The listing builds one solid part. Answer for the finished solid, in the listing's coordinates (mm). Face numbers are marked on the shaded views. A direction names the side the tool comes from. Coordinates: 2 decimals unless noted, no trailing zeros. Loops run counter-clockwise (first coordinate to the right, second up) from the corner with the lowest first, then second, coordinate; pieces in that order, holes last. Notation, with made-up numbers: (30.25, 26.5) - (76.25, 26.5) arc R15 ccw to (76.25, 34.5) - close; hole circle Ø5 at (56.5, 89.5). An arc over 180 degrees is marked (long way). Return JSON: item names as keys, results as strings. Group by question number.
1. The mould has two halves that part along X. Classify the marked faces 3, 4, 5 and 6: pulls with the +X half, pulls with the -X half, needs draft (parallel to the pull), parting line crosses it, or undercut.
2. Each of these flat-tipped pins is pushed along its axis until it touches: P1, Ø7.5, axis at x = -8, z = 12, coming from the -Y side; P2, Ø1.5, axis at x = 9, y = 2.5, coming from the -Z side; P3, Ø7, axis at x = 0, z = 0, coming from the -Y side; P4, Ø4, axis at y = 1.5, z = 8.5, coming from the +X side. Where does it stop, or does it pass through?
3. Section D-D (z = -10.16) is taken. Write down the section's boundary in (x, y) (3 decimals), and give its area (3 significant figures).
4. Find the intervals of material crossed by line 1 along X through (y, z) = (4, 0) (3 decimals); line 2 along X through (y, z) = (4.5, 7); line 3 along Z through (x, y) = (1, 7.25), in increasing order.
5. Section B-B (y = 2.5) is taken. Write down the section's boundary in (x, z) (3 decimals), and give its area (3 significant figures).
6. Which of the six approach directions +Z, -Z, +X, -X, +Y, -Y give full straight-line access (tool end or side, diameter ignored) to the marked faces 1 and 2?
7. Section C-C (x = 0) is taken. Write down the section's boundary in (y, z) (3 decimals), and give its area (3 significant figures).
8. Section A-A (z = 0) is taken. Write down the section's boundary in (x, y) (3 decimals).
Autodesk Inventor part; units mm, degrees
ref_plane "YZ Plane" through (0, 0, 0) normal (1, 0, 0) x (0, 1, 0)
ref_plane "XZ Plane" through (0, 0, 0) normal (0, 1, 0) x (-1, 0, 0)
ref_plane "XY Plane" through (0, 0, 0) normal (0, 0, 1) x (1, 0, 0)
sketch "Sketch1" plane through (0, 0, 0) normal (0, 1, 0) x (-1, 0, 0)
  circle A0 centre (0, 0) radius 3.81
  circle A1 centre (0, 0) radius 16.51
  line L0 (0, 0) -> (10.16, 0)
  line L1 (0, 0) -> (-10.16, 0)
  circle A2 centre (10.16, 0) radius 1.524
  circle A3 centre (-10.16, 0) radius 1.524
  circle A4 centre (0, 0) radius 5.0292
  circle A5 centre (0, 0) radius 15.2908
  line L2 (0, 0) -> (0, 10.16)
  circle A6 centre (0, 10.16) radius 2.3812
  line L3 (0, 0) -> (2.5146, 4.3554)
  line L4 (0, 0) -> (5.0292, 0) construction
  line L5 (2.5146, 4.3554) -> (7.6454, 13.2422)
  line L6 (0, 0) -> (-2.5146, 4.3554)
  line L7 (-2.5146, 4.3554) -> (-7.6454, 13.2422)
  line L8 (0, 0) -> (2.5146, -4.3554)
  line L9 (2.5146, -4.3554) -> (7.6454, -13.2422)
  line L10 (0, 0) -> (-2.5146, -4.3554)
  line L11 (-2.5146, -4.3554) -> (-7.6454, -13.2422)
  line L12 (0.4064, 16.8443) -> (-0.4064, 16.8443)
  line L13 (-0.4064, 16.8443) -> (-0.4064, 15.0672)
  line L14 (-0.4064, 15.0672) -> (0.4064, 15.0672)
  line L15 (0.4064, 15.0672) -> (0.4064, 16.8443)
  line L16 (0.4064, 16.8443) -> (-0.4064, 15.0672) construction
  line L17 (-0.4064, 16.8443) -> (0.4064, 15.0672) construction
  line L18 (0.4064, -15.0362) -> (-0.4064, -15.0362)
  line L19 (-0.4064, -15.0362) -> (-0.4064, -16.8142)
  line L20 (-0.4064, -16.8142) -> (0.4064, -16.8142)
  line L21 (0.4064, -16.8142) -> (0.4064, -15.0362)
  line L22 (0.4064, -15.0362) -> (-0.4064, -16.8142) construction
  line L23 (-0.4064, -15.0362) -> (0.4064, -16.8142) construction
  circle A7 centre (0, 10.16) radius 1.524
  line L24 (0, 0) -> (0, -10.16)
  circle A8 centre (0, -10.16) radius 1.524
  circle A9 centre (0, 0) radius 0.7937
  line L25 (0, 0) -> (-13.5242, 9.4697)
  line L26 (0, 0) -> (16.51, 0) construction
  line L27 (-13.9904, 8.8039) -> (-0.408, -0.7066)
  line L28 (-13.058, 10.1356) -> (0.2563, 0.8128)
  line L29 (16.49, 0.8128) -> (16.51, 0.8128)
  line L30 (16.49, -0.8128) -> (16.51, -0.8128)
  line L31 (0, 0) -> (-0.408, -0.7066)
  line L32 (0.2563, 0.8128) -> (0.408, 0.7066)
  line L33 (0, 0) -> (0.408, 0.7066)
  line L34 (-13.058, 10.1356) -> (-13.9904, 8.8039)
  line L35 (0.408, 0.7066) -> (-0.408, -0.7066)
  line L36 (-7.6454, 13.2422) -> (-8.255, 14.2981)
  line L37 (7.6454, 13.2422) -> (8.255, 14.2981)
  line L38 (-7.6454, -13.2422) -> (-8.255, -14.2981)
  line L39 (7.6454, -13.2422) -> (8.255, -14.2981)
  line L40 (0, 0) -> (13.2422, 7.6454)
  line L41 (13.2422, 7.6454) -> (14.2981, 8.255)
  line L42 (0, 0) -> (-13.2422, -7.6454)
  line L43 (-13.2422, -7.6454) -> (-14.2981, -8.255)
  point P0 (0, 15.9557)
  point P1 (0, -15.9252)
  point P2 (-13.974, 8.7925)
  point P3 (-1.4171, 0)
  point P4 (-0.7937, 0)
  point P5 (-0.3969, 0.6874)
  point P6 (-0.9616, 1.6656)
  point P7 (-13.0416, 10.1241)
  point P8 (1.905, 3.2996)
  point P9 (-1.905, 3.2996)
  point P10 (1.905, -3.2996)
  point P11 (-1.905, -3.2996)
  point P12 (4.3554, 2.5146)
  point P13 (-4.3554, -2.5146)
  point P14 (3.2996, 1.905)
  point P15 (-3.2996, -1.905)
  dimension "d1" = 33.02
  dimension "d0" = 7.62
  dimension "d2" = 10.16
  dimension "d3" = 10.16
  dimension "d4" = 3.048
  dimension "d5" = 3.048
  dimension "d8" = 10.0584
  dimension "d9" = 30.5816
  dimension "d10" = 10.16
  dimension "d11" = 4.7625
  dimension "d12" = 60
  dimension "d17" = 0.8128
  dimension "d18" = 0.8128
  dimension "d19" = 1.778
  dimension "d24" = 3.048
  dimension "d25" = 10.16
  dimension "d26" = 3.048
  dimension "d41" = 1.5875
  dimension "d42" = 145
  dimension "d43" = 0.8128
  dimension "d44" = 0.8128
extrude "Extrusion1" add sketch "Sketch1" along normal blind 7.5184 contours L0 A4 L8 A0 | A0 L40 A4 L0 | A0 L3 A4 L40 | L8 A4 L24 A0 | A2 | A4 L40 A5 L9 | A0 L2 A4 L3 | A4 L5 A5 L40 | L24 A4 L10 A0 | A8 | L9 A5 L21 L18 L19 L11 A4 | A0 L6 A4 L2 | A7 | A6 | A4 L7 A5 L13 L14 L15 L5 | L41 A1 L39 A5 | A5 L37 A1 L41 | L10 A4 L42 A0 | L39 A1 L21 A5 | A0 L28 A4 L6 | A5 L15 A1 L37 | L42 A4 L1 A0 | L11 A5 L42 A4 | L21 A1 L19 A5 | A5 L19 L18 L21 | L25 A4 L28 A0 | A0 L27 A4 L25 | A4 L28 A5 L7 | L15 L14 L13 A5 | A5 L13 A1 L15 | L1 A4 L27 A0 | A3 | L42 A5 L27 A4 | L38 A1 L43 A5 | A5 L19 A1 L38 | L25 A5 L28 A4 | A4 L27 A5 L25 | L36 A1 L13 A5 | A5 L28 A1 L36 | L43 A1 L27 A5 | L25 A1 L28 A5 | A5 L27 A1 L25
extrude "Extrusion2" cut sketch "Sketch1" along normal blind 6.35 contours A0 L3 A4 L40 | A0 L2 A4 L3 | A4 L5 A5 L40 | A0 L6 A4 L2 | A7 | A6 | A4 L7 A5 L13 L14 L15 L5 | A5 L37 A1 L41 | A5 L15 A1 L37 | L15 L14 L13 A5 | A5 L13 A1 L15 | L36 A1 L13 A5
extrude "Extrusion3" cut sketch "Sketch1" along normal blind 6.35 contours L8 A4 L24 A0 | L24 A4 L10 A0 | A8 | L9 A5 L21 L18 L19 L11 A4 | L10 A4 L42 A0 | L39 A1 L21 A5 | L11 A5 L42 A4 | L21 A1 L19 A5 | A5 L19 L18 L21 | L38 A1 L43 A5 | A5 L19 A1 L38
extrude "Extrusion6" cut sketch "Sketch1" along normal blind 7.5184 contours L1 L27 A0 L25 A9 | A9 L25 A0 L28 L6 | L25 A4 L28 A0 | A0 L27 A4 L25 | L25 A5 L28 A4 | A4 L27 A5 L25 | L25 A1 L28 A5 | A5 L27 A1 L25
hole "Hole3" at (10.16, 0, 0) direction (0, 1, 0) diameter 3.81 end through all
hole "Hole4" at (-10.16, 0, 0) direction (0, 1, 0) diameter 3.81 end through all
hole "Hole5" at (0, 0, -10.16) direction (0, 1, 0) diameter 3.81 end through all
hole "Hole6" at (0, 0, 10.16) direction (0, 1, 0) diameter 3.81 end through all
properties part number "tab3"
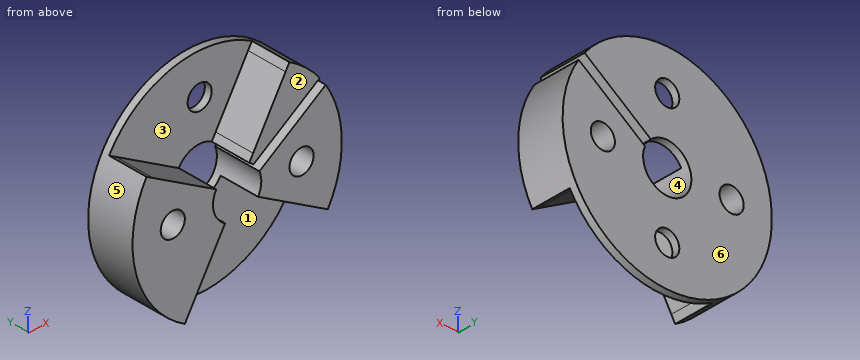
The answers:
{
 "1": {"face 3": "undercut", "face 4": "undercut", "face 5": "parting line crosses it", "face 6": "needs draft"},
 "2": {"P1": "stops at y = 6.35", "P2": "stops at z = -5.63", "P3": "passes through", "P4": "stops at x = 15.18"},
 "3": {"outline": "(-13.014, 0) - (-5.866, 0) - (-5.866, 6.35) - (-1.905, 6.35) - (-1.905, 7.518) - (-13.014, 7.518) - close; (1.905, 6.35) - (13.014, 6.35) - (13.014, 7.518) - (1.905, 7.518) - close", "area": "71.3 mm2"},
 "4": {"line 1": "x = -16.51 to -12.065, -8.255 to -3.81, 3.81 to 8.255, 12.065 to 16.51", "line 2": "x = -14.95 to -12.12, 4.04 to 8.58, 11.41 to 14.95", "line 3": "z = -16.48 to -11.78, -8.54 to -3.68, 3.68 to 8.54, 11.78 to 16.48"},
 "5": {"outline": "(-14.298, 8.255) arc R16.51 ccw to (-8.255, -14.298) - (-7.645, -13.242) - (-2.515, -4.355) - (-1.905, -3.3) arc R3.81 cw to (-3.3, 1.905) - (-13.242, 7.645) - close; (1.905, 3.3) arc R3.81 cw to (2.583, 2.801) - (13.042, 10.124) arc R16.51 ccw to (8.255, 14.298) - (7.645, 13.242) - (2.515, 4.355) - close; (3.3, -1.905) - (13.242, -7.645) - (14.298, -8.255) arc R16.51 ccw to (13.974, 8.792) - (3.515, 1.469) arc R3.81 cw to start; hole circle Ø3.81 at (-10.16, 0); hole circle Ø3.81 at (10.16, 0)", "area": "362 mm2"},
 "6": {"face 1": "-Z, -Y", "face 2": "+Z, -Z, +X, -X, -Y"},
 "7": {"outline": "(6.35, -16.51) - (7.518, -16.51) - (7.518, -12.065) - (6.35, -12.065) - close; (6.35, -8.255) - (7.518, -8.255) - (7.518, -3.81) - (6.35, -3.81) - close; (6.35, 3.81) - (7.518, 3.81) - (7.518, 8.255) - (6.35, 8.255) - close; (6.35, 12.065) - (7.518, 12.065) - (7.518, 16.51) - (6.35, 16.51) - close", "area": "20.8 mm2"},
 "8": {"outline": "(-16.51, 0) - (-12.065, 0) - (-12.065, 7.518) - (-16.51, 7.518) - close; (-8.255, 0) - (-3.81, 0) - (-3.81, 7.518) - (-8.255, 7.518) - close; (3.81, 0) - (8.255, 0) - (8.255, 7.518) - (3.81, 7.518) - close; (12.065, 0) - (16.51, 0) - (16.51, 7.518) - (12.065, 7.518) - close"}
}
